from build123d import *

# Parameters (mm, degrees)
SKETCH1_R               = 5
BOSS_EXTRUDE1_DEPTH     = 152
CUT_EXTRUDE2_DEPTH      = 153.164384795
CUT_EXTRUDE2_DEPTH_BACK = 153.164384795
SKETCH3_R               = 2.05
SKETCH5_W               = 15
SKETCH5_H               = 2
CUT_EXTRUDE4_DEPTH      = 50
SKETCH6_OUTSIDE_W       = 42.532
SKETCH6_OUTSIDE_H       = 42.532
SKETCH6_OUTSIDE_R       = 4
CUT_EXTRUDE5_DEPTH      = 20


with BuildPart() as part:
    # Sketch1 → Boss-Extrude1 (new body)
    with BuildSketch(Plane.XY):
        Circle(SKETCH1_R)
    extrude(amount=BOSS_EXTRUDE1_DEPTH)

    # Sketch3 → Cut-Extrude2 (cut, two sides: drawn at the far end of the back side and taken through both)
    with BuildSketch(Plane(origin=(0, 0, 0), x_dir=(1, 0, 0), z_dir=(0, 1, 0)).offset(-CUT_EXTRUDE2_DEPTH_BACK)):
        with Locations(Location((0, -10, 0), (0, 0, 270))):
            Circle(SKETCH3_R)
        with Locations(Location((0, -35, 0), (0, 0, 270))):
            Circle(SKETCH3_R)
    extrude(amount=CUT_EXTRUDE2_DEPTH + CUT_EXTRUDE2_DEPTH_BACK, mode=Mode.SUBTRACT)

    # Sketch5 → Cut-Extrude4 (cut)
    with BuildSketch(Plane(origin=(0, 0, 0), x_dir=(-1, 0, 0), z_dir=(0, 0, -1))):
        Rectangle(SKETCH5_W, SKETCH5_H)
    extrude(amount=-CUT_EXTRUDE4_DEPTH, mode=Mode.SUBTRACT)

    # Sketch6 outside → Cut-Extrude5 (cut)
    with BuildSketch(Plane.XY.offset(152)):
        Rectangle(SKETCH6_OUTSIDE_W, SKETCH6_OUTSIDE_H)
        Circle(SKETCH6_OUTSIDE_R, mode=Mode.SUBTRACT)
    extrude(amount=-CUT_EXTRUDE5_DEPTH, mode=Mode.SUBTRACT)


solid = part.part
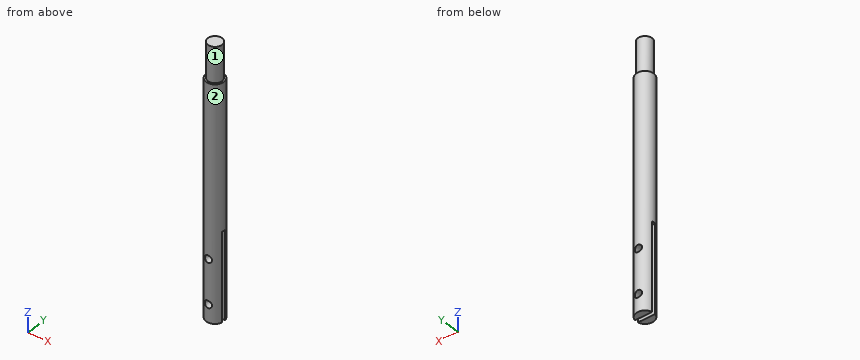
Source: CAD feature listing. Evaluate the final solid. Frame: model axes, mm. Face numbers are marked on the shaded views. A direction names the side the tool comes from. Round coordinates to 2 decimals unless told otherwise and drop trailing zeros. Loops run counter-clockwise (first coordinate to the right, second up) from the corner with the lowest first, then second, coordinate; pieces in that order, holes last. Notation, with made-up numbers: (36.25, -20.75) - (91.25, -20.75) arc R22 cw to (91.25, -12.75) - close; hole circle Ø11 at (-8, -8.5). An arc over 180 degrees is marked (long way). Write item = value, one per line. Start each with the question number.
Item 1: Material intervals for line 1 (Z direction, x = 0, y = 2.3); line 2 (Y direction, x = -3, z = 113.5); line 3 (Y direction, x = -0.5, z = 116), sorted ascending.
Item 2: Reachability of the marked faces 1 and 2 from +Z, -Z, +X, -X, +Y, -Y: full face, straight path, thin tool, end or side. Return the list, or none.
Item 3: Section query D-D on z = 142. Output: boundary loops of the cut face in (x, y).
Item 4: First-contact query: pin 1 Ø2.5 at (x, z) = (0, 10) entering from -Y; pin 2 Ø1 at (x, y) = (2, 0) entering from -Z; pin 3 Ø2 at (x, z) = (3, 115) entering from -Y; pin 4 Ø5 at (y, z) = (-3.5, 132) entering from -X. Flat tips, straight axial feed; report the tip coordinate or a pass-through.
Item 5: Section query B-B on z = 39.5. Output: boundary loops of the cut face in (x, y), plus the area to 3 significant figures.
Item 6: Section query A-A on z = 10. Output: boundary loops of the cut face in (x, y).
Item 7: Section query C-C on z = 114. Output: boundary loops of the cut face in (x, y), plus the area to 3 significant figures.
Results list:
q1.line_1 = 0 to 7.95, 12.05 to 32.95, 37.05 to 152
q1.line_2 = -4 to 4
q1.line_3 = -4.97 to 4.97
q2.face_1 = +Z
q2.face_2 = +Z, -Z
q3.outline = circle Ø8 at (0, 0)
q4.pin_1 = through
q4.pin_2 = 50
q4.pin_3 = -4.58
q4.pin_4 = -4.9
q5.outline = (-4.9, -1) arc R5 ccw to (4.9, -1) - close; (-4.9, 1) - (4.9, 1) arc R5 ccw to start
q5.area = 58.7 mm²
q6.outline = (-4.9, -1) arc R5 ccw to (-2.05, -4.56) - (-2.05, -1) - close; (-4.9, 1) - (-2.05, 1) - (-2.05, 4.56) arc R5 ccw to start; (2.05, -4.56) arc R5 ccw to (4.9, -1) - (2.05, -1) - close; (2.05, 1) - (4.9, 1) arc R5 ccw to (2.05, 4.56) - close
q7.outline = circle Ø10 at (0, 0)
q7.area = 78.5 mm²
